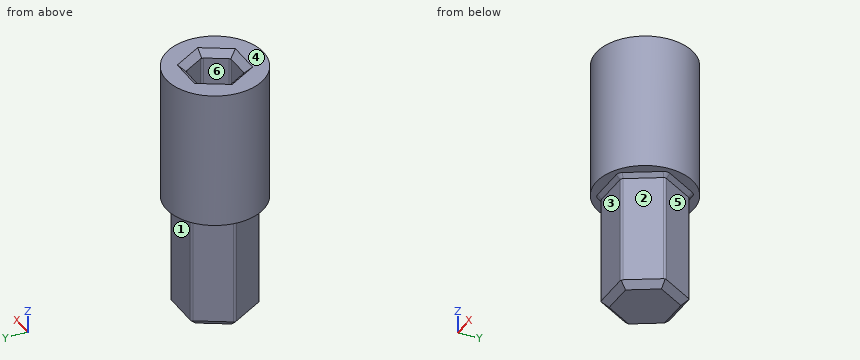
Autodesk Fusion 360 part; units mm, degrees
sketch "Sketch1" plane through (0, 0, 0) normal (0, 0, 1) x (1, 0, 0)
  line L0 (3.8275, 0) -> (1.9137, 3.3147)
  line L1 (1.9137, 3.3147) -> (-1.9137, 3.3147)
  line L2 (-1.9137, 3.3147) -> (-3.8275, 0)
  line L3 (-3.8275, 0) -> (-1.9137, -3.3147)
  line L4 (-1.9137, -3.3147) -> (1.9137, -3.3147)
  line L5 (1.9137, -3.3147) -> (3.8275, 0)
  line L6 (0, 0) -> (0, -3.3147) construction
  dimension "d1" = 6.6294
extrude "Extrude1" add sketch "Sketch1" along normal blind 11.43
sketch "Sketch2" plane through (0, 0, 11.43) normal (0, 0, 1) x (-1, 0, 0)
  line L0 (-1.9137, 3.3147) -> (-3.8275, 0)
  line L1 (-3.8275, 0) -> (-1.9137, -3.3147)
  line L2 (-1.9137, -3.3147) -> (1.9137, -3.3147)
  line L3 (1.9137, -3.3147) -> (3.8275, 0)
  line L4 (3.8275, 0) -> (1.9137, 3.3147)
  line L5 (1.9137, 3.3147) -> (-1.9137, 3.3147)
  line L6 (-2.515, 0) -> (-1.2575, -2.1781)
  line L7 (-1.2575, -2.1781) -> (1.2575, -2.1781)
  line L8 (1.2575, -2.1781) -> (2.515, 0)
  line L9 (2.515, 0) -> (1.2575, 2.1781)
  line L10 (1.2575, 2.1781) -> (-1.2575, 2.1781)
  line L11 (-1.2575, 2.1781) -> (-2.515, 0)
  line L12 (0, 2.1781) -> (0, 0) construction
  line L13 (-2.724, 4.7181) -> (-5.4479, 0) construction
  line L14 (-5.4479, 0) -> (-2.724, -4.718) construction
  line L15 (-2.724, -4.718) -> (2.724, -4.718) construction
  line L16 (2.724, -4.718) -> (5.4479, 0) construction
  line L17 (5.4479, 0) -> (2.724, 4.7181) construction
  line L18 (2.724, 4.7181) -> (-2.724, 4.7181) construction
  circle A0 centre (0, 0) radius 4.7181
  dimension "d5" = 4.3561
  dimension "d6" = 2.54
extrude "Extrude2" add sketch "Sketch2" along normal blind 13.335 contours L0 L1 L2 L3 L4 L5 | A0
chamfer "Chamfer1" distance 0.635 angle 45 6 edges at (0, -2.1781, 24.765) (-1.8862, -1.089, 24.765) (-1.8862, 1.089, 24.765) (0, 2.1781, 24.765) (1.8862, 1.089, 24.765) (1.8862, -1.089, 24.765) 1 faces at (1.2758, 0, 0)
fillet "Fillet1" radius 0.2858 12 edges at (-3.8275, 0, 6.0325) (-1.9137, -3.3147, 6.0325) (1.9137, -3.3147, 6.0325) (-1.9137, 3.3147, 6.0325) (1.9137, 3.3147, 6.0325) (3.8275, 0, 6.0325) (2.515, 0, 17.78) (1.2575, -2.1781, 17.78) (-1.2575, -2.1781, 17.78) (-2.515, 0, 17.78) (-1.2575, 2.1781, 17.78) (1.2575, 2.1781, 17.78)
chamfer "Chamfer2" distance 0.381 angle 45 12 edges at (2.8706, 1.6574, 11.43) (1.8916, 3.2764, 11.43) (0, 3.3147, 11.43) (-1.8916, 3.2764, 11.43) (-2.8706, 1.6574, 11.43) (-3.7833, 0, 11.43) (-2.8706, -1.6574, 11.43) (-1.8916, -3.2764, 11.43) (0, -3.3147, 11.43) (1.8916, -3.2764, 11.43) (2.8706, -1.6574, 11.43) (3.7833, 0, 11.43)
chamfer "Chamfer3" distance 0.2223 angle 45 1 faces at (0.3642, 0.726, 11.43)
equation "d1 = 0.248 in + 0.013 in"
equation "d5 = 0.1565 in + ( 0.015 ) * 1 in"
Source: CAD feature listing. Evaluate the final solid. Frame: model axes, mm. Face numbers are marked on the shaded views. A direction names the side the tool comes from. Give positions to 0.01 mm unless a question says otherwise; leave off trailing zeros. Order: outer loops, then holes, each group sorted by start corner. A loop starts at its lowest first (then second) coordinate and runs counter-clockwise, first axis right, second up. Notation, with made-up numbers: (14, 85) -> (68, 85) arc R38 cw to (68, 124) -> close; hole circle Ø6 at (34.25, -7). An arc over 180 degrees is marked (long way). Use a Markdown table: item, result.
1) Section query B-B, the plane z = 18.5. Return the cut outline in (x, y), then the cut area to 3 significant figures.
Answer list:
| item | result |
|---|---|
| outline | circle Ø9.44 at (0, 0); hole (-2.43, -0.14) -> (-1.34, -2.04) arc R0.29 ccw to (-1.09, -2.18) -> (1.09, -2.18) arc R0.29 ccw to (1.34, -2.04) -> (2.43, -0.14) arc R0.29 ccw to (2.43, 0.14) -> (1.34, 2.04) arc R0.29 ccw to (1.09, 2.18) -> (-1.09, 2.18) arc R0.29 ccw to (-1.34, 2.04) -> (-2.43, 0.14) arc R0.29 ccw to start |
| area | 53.5 mm² |
2) Reachability of the marked faces 1, 2 and 3 from +Z, -Z, +X, -X, +Y, -Y: full face, straight path, thin tool, end or side. Return the list, or none.
Answer list:
| item | result |
|---|---|
| face 1 | -Z, +X, -X, +Y |
| face 2 | -Z, +X, -Y |
| face 3 | -Z, +X, -X, -Y |
3) Contact query for flat-ended pins moving along their axis: P1, Ø1, axis at x = -0.5, z = 4.5, coming from the +Y side; P2, Ø4, axis at x = 0.5, z = 8, coming from the -Y side; P3, Ø1.2, axis at x = -1, y = -0.5, coming from the +Z side. Output: stop coordinate, or through.
Answer list:
| item | result |
|---|---|
| P1 | y = 3.31 |
| P2 | y = -3.31 |
| P3 | z = 11.43 |
4) Section query D-D, the plane y = -1. Return the cut outline in (x, z) (3 decimals), then the cut area to 3 significant figures.
Answer list:
| item | result |
|---|---|
| outline | (-4.611, 11.43) -> (-3.69, 11.43) -> (-3.25, 11.049) -> (-3.25, 0.635) -> (-2.517, 0) -> (2.517, 0) -> (3.25, 0.635) -> (3.25, 11.049) -> (3.69, 11.43) -> (4.611, 11.43) -> (4.611, 24.765) -> (2.671, 24.765) -> (1.938, 24.13) -> (1.938, 11.652) -> (1.681, 11.43) -> (-1.681, 11.43) -> (-1.938, 11.652) -> (-1.938, 24.13) -> (-2.671, 24.765) -> (-4.611, 24.765) -> close |
| area | 145 mm² |
5) Section query A-A, the plane z = 3. Return the cut outline in (x, y) (3 decimals).
Answer list:
| item | result |
|---|---|
| outline | (-3.745, -0.143) -> (-1.996, -3.172) arc R0.286 ccw to (-1.749, -3.315) -> (1.749, -3.315) arc R0.286 ccw to (1.996, -3.172) -> (3.745, -0.143) arc R0.286 ccw to (3.745, 0.143) -> (1.996, 3.172) arc R0.286 ccw to (1.749, 3.315) -> (-1.749, 3.315) arc R0.286 ccw to (-1.996, 3.172) -> (-3.745, 0.143) arc R0.286 ccw to start |
6) Mould query, pull axis X, two halves, no side actions, for the marked faces 4, 5 and 6. Classes: +X half, -X half, draft (parallel to the pull), parting line (faces both ways), or undercut.
Answer list:
| item | result |
|---|---|
| face 4 | draft |
| face 5 | +X half |
| face 6 | undercut |
7) Ray query, line 1 along Z through (x, y) = (-2.75, -3.5) (3 decimals); line 2 along Y through (x, z) = (-2.25, 12.5); line 3 along Y through (x, z) = (1.75, 9.75). Return the intervals inside material, ascending. Write a range as [from, to].
Answer list:
| item | result |
|---|---|
| line 1 | [11.43, 24.765] |
| line 2 | [-4.15, -0.46], [0.46, 4.15] |
| line 3 | [-3.31, 3.31] |
8) Section query C-C, the plane x = 0. Return the cut outline in (y, z) (3 decimals), then the cut area to 3 significant figures.
Answer list:
| item | result |
|---|---|
| outline | (-4.718, 11.43) -> (-3.696, 11.43) -> (-3.315, 11.049) -> (-3.315, 0.635) -> (-2.68, 0) -> (2.68, 0) -> (3.315, 0.635) -> (3.315, 11.049) -> (3.696, 11.43) -> (4.718, 11.43) -> (4.718, 24.765) -> (2.813, 24.765) -> (2.178, 24.13) -> (2.178, 11.652) -> (1.956, 11.43) -> (-1.956, 11.43) -> (-2.178, 11.652) -> (-2.178, 24.13) -> (-2.813, 24.765) -> (-4.718, 24.765) -> close |
| area | 143 mm² |
